The model under review builds one solid part; all positions refer to its coordinate system, in mm. A direction names the side the tool comes from. Round coordinates to 2 decimals unless told otherwise and drop trailing zeros. Loops run counter-clockwise (first coordinate to the right, second up) from the corner with the lowest first, then second, coordinate; pieces in that order, holes last. Notation, with made-up numbers: M 69,-12 L 117,-12 A13 ccw 117,-1 Z; hole C -34,17 d6. An arc over 180 degrees is marked long. Answer as a JSON object with one key per item and string values. Group by question number.
Item 1: Tool access review of faces 4 (the face through (47, 16, 10)), 5 (the face through (47.2, 18.1, -21.15)), 6 (the face through (-47.2, 18.1, 21.15)): name each direction out of +Z, -Z, +X, -X, +Y, -Y from which nothing blocks a thin tool from reaching the whole face with its end or side.
Item 2: Consider section A-A (y = 26.15). Give the boundary of the cut face in (x, z).
Item 3: Consider section C-C (z = 23). Give the boundary of the cut face in (x, y), and give its area (3 significant figures).
Item 4: Consider section B-B (x = 18.5). Give the boundary of the cut face in (y, z).
Item 5: To check wall thickness, follow line 1 (X direction, y = 15, z = 20); line 2 (Y direction, x = -48.1, z = 15.5); line 3 (X direction, y = 2, z = 0). State the ranges of each line that lie inside material, in increasing order.
Item 6: Insertion check: P1, Ø2.5, axis at y = 41.65, z = 15.5, coming from the -X side; P2, Ø8, axis at x = -44, y = 22.5, coming from the -Z side. Each pin has a flat end and moves straight along its axis. Give the tip position at first contact, or say it passes through.
Item 7: Consider section D-D (y = 41.65). Give the boundary of the cut face in (x, z), and give its area (3 significant figures).
Item 8: The part is to be moulded in two halves that separate along Z. For faces 1 (the face through (-47.2, 18.1, -21.15)), 2 (the face through (48, 18, 21.15)), 3 (the face through (-48.5, 41.7, -17.1)), say which applies: +Z half, -Z half, draft (parallel to the pull), parting line (faces both ways), or undercut.
```python
from build123d import *

# Parameters (mm, degrees)
BODY_DEPTH                = 5
SKETCH4_W                 = 3
SKETCH4_H                 = 42.3
EXTRUDE_WING_DEPTH        = 42.3
SKETCH5_R                 = 1.6
SKETCH5_R_2               = 13.5
CUT_MOTOR_HOLES_DEPTH     = 120.424829914
CUT_EXCESS_MATERIAL_REACH = 84.233
SKETCH8_R                 = 30
CUT_DECK_HOLES_REACH      = 81.463
SKETCH9_R                 = 1.6


with BuildPart() as part:
    # Sketch1 → body (new body)
    with BuildSketch(Plane(origin=(0, 0, 0), x_dir=(1, 0, 0), z_dir=(0, 1, 0))):
        with BuildLine():
            Line((-39.719988671, 21.15), (-50, 21.15))
            Line((-50, 21.15), (-50, -21.15))
            Line((-50, -21.15), (-39.719988671, -21.15))
            ThreePointArc((-39.719988671, -21.15), (0, -45), (39.719988671, -21.15))
            Line((39.719988671, -21.15), (50, -21.15))
            Line((50, -21.15), (50, 21.15))
            Line((50, 21.15), (39.719988671, 21.15))
            ThreePointArc((39.719988671, 21.15), (0, 45), (-39.719988671, 21.15))
        make_face()
    extrude(amount=BODY_DEPTH)

    # Sketch4 → extrude-wing (add)
    with BuildSketch(Plane(origin=(0, 5, 0), x_dir=(1, 0, 0), z_dir=(0, 1, 0))):
        with Locations((-48.5, 0)):
            Rectangle(SKETCH4_W, SKETCH4_H)
        with Locations((48.5, 0)):
            Rectangle(SKETCH4_W, SKETCH4_H)
    extrude(amount=EXTRUDE_WING_DEPTH)

    # Sketch5 → cut-motor-holes (cut, through all)
    with BuildSketch(Plane.ZY.offset(50)):
        with Locations((-15.5, 41.65)):
            Circle(SKETCH5_R)
        with Locations((15.5, 41.65)):
            Circle(SKETCH5_R)
        with Locations((15.5, 10.65)):
            Circle(SKETCH5_R)
        with Locations((-15.5, 10.65)):
            Circle(SKETCH5_R)
        with Locations((0, 26.15)):
            Circle(SKETCH5_R_2)
    extrude(amount=-CUT_MOTOR_HOLES_DEPTH, mode=Mode.SUBTRACT)

    # Sketch8 → cut-excess-material (cut, up to next)
    with BuildSketch(Plane.XZ, mode=Mode.PRIVATE) as cut_excess_material_sk1:
        with Locations(Location((0, 0, 0), (0, 0, 270))):
            Circle(SKETCH8_R)
    cut_excess_material_tool1 = extrude(cut_excess_material_sk1.sketch, amount=-CUT_EXCESS_MATERIAL_REACH, mode=Mode.PRIVATE) & part.part
    add(cut_excess_material_tool1.solids().sort_by_distance((0, 0, 0))[0], mode=Mode.SUBTRACT)

    # Sketch9 → cut-deck-holes (cut, up to next)
    with BuildSketch(Plane(origin=(0, 5, 0), x_dir=(1, 0, 0), z_dir=(0, 1, 0)), mode=Mode.PRIVATE) as cut_deck_holes_sk1:
        with Locations(Location((44, -17.5, 0), (0, 0, 270))):
            Circle(SKETCH9_R)
    cut_deck_holes_tool1 = extrude(cut_deck_holes_sk1.sketch, amount=-CUT_DECK_HOLES_REACH, mode=Mode.PRIVATE) & part.part
    # Sketch9 → cut-deck-holes (cut, up to next)
    with BuildSketch(Plane(origin=(0, 5, 0), x_dir=(1, 0, 0), z_dir=(0, 1, 0)), mode=Mode.PRIVATE) as cut_deck_holes_sk2:
        with Locations(Location((44, 17.5, 0), (0, 0, 270))):
            Circle(SKETCH9_R)
    cut_deck_holes_tool2 = extrude(cut_deck_holes_sk2.sketch, amount=-CUT_DECK_HOLES_REACH, mode=Mode.PRIVATE) & part.part
    # Sketch9 → cut-deck-holes (cut, up to next)
    with BuildSketch(Plane(origin=(0, 5, 0), x_dir=(1, 0, 0), z_dir=(0, 1, 0)), mode=Mode.PRIVATE) as cut_deck_holes_sk3:
        with Locations(Location((-44, 17.5, 0), (0, 0, 270))):
            Circle(SKETCH9_R)
    cut_deck_holes_tool3 = extrude(cut_deck_holes_sk3.sketch, amount=-CUT_DECK_HOLES_REACH, mode=Mode.PRIVATE) & part.part
    # Sketch9 → cut-deck-holes (cut, up to next)
    with BuildSketch(Plane(origin=(0, 5, 0), x_dir=(1, 0, 0), z_dir=(0, 1, 0)), mode=Mode.PRIVATE) as cut_deck_holes_sk4:
        with Locations(Location((-44, -17.5, 0), (0, 0, 270))):
            Circle(SKETCH9_R)
    cut_deck_holes_tool4 = extrude(cut_deck_holes_sk4.sketch, amount=-CUT_DECK_HOLES_REACH, mode=Mode.PRIVATE) & part.part
    add(cut_deck_holes_tool1.solids().sort_by_distance((44, 5, 17.5))[0], mode=Mode.SUBTRACT)
    add(cut_deck_holes_tool2.solids().sort_by_distance((44, 5, -17.5))[0], mode=Mode.SUBTRACT)
    add(cut_deck_holes_tool3.solids().sort_by_distance((-44, 5, -17.5))[0], mode=Mode.SUBTRACT)
    add(cut_deck_holes_tool4.solids().sort_by_distance((-44, 5, 17.5))[0], mode=Mode.SUBTRACT)


solid = part.part
```
Geometry results:
{
 "1": {"face 4": "+Z, -Z, +Y", "face 5": "-Z, +X, +Y, -Y", "face 6": "+Z, -X, +Y, -Y"},
 "2": {"outline": "M -50,-21.15 L -47,-21.15 L -47,-13.5 L -50,-13.5 Z; M -50,13.5 L -47,13.5 L -47,21.15 L -50,21.15 Z; M 47,-21.15 L 50,-21.15 L 50,-13.5 L 47,-13.5 Z; M 47,13.5 L 50,13.5 L 50,21.15 L 47,21.15 Z"},
 "3": {"outline": "M -38.68,0 L -19.26,0 L -19.26,5 L -38.68,5 Z; M 19.26,0 L 38.68,0 L 38.68,5 L 19.26,5 Z", "area": "194 mm^2"},
 "4": {"outline": "M 0,-41.02 L 5,-41.02 L 5,-23.62 L 0,-23.62 Z; M 0,23.62 L 5,23.62 L 5,41.02 L 0,41.02 Z"},
 "5": {"line 1": "x = -50 to -47, 47 to 50", "line 2": "y = 0 to 9.05, 12.25 to 40.05, 43.25 to 47.3", "line 3": "x = -50 to -30, 30 to 50"},
 "6": {"P1": "passes through", "P2": "stops at z = -21.15"},
 "7": {"outline": "M -50,-21.15 L -47,-21.15 L -47,-17.1 L -50,-17.1 Z; M -50,-13.9 L -47,-13.9 L -47,13.9 L -50,13.9 Z; M -50,17.1 L -47,17.1 L -47,21.15 L -50,21.15 Z; M 47,-21.15 L 50,-21.15 L 50,-17.1 L 47,-17.1 Z; M 47,-13.9 L 50,-13.9 L 50,13.9 L 47,13.9 Z; M 47,17.1 L 50,17.1 L 50,21.15 L 47,21.15 Z", "area": "215 mm^2"},
 "8": {"face 1": "-Z half", "face 2": "+Z half", "face 3": "undercut"}
}
